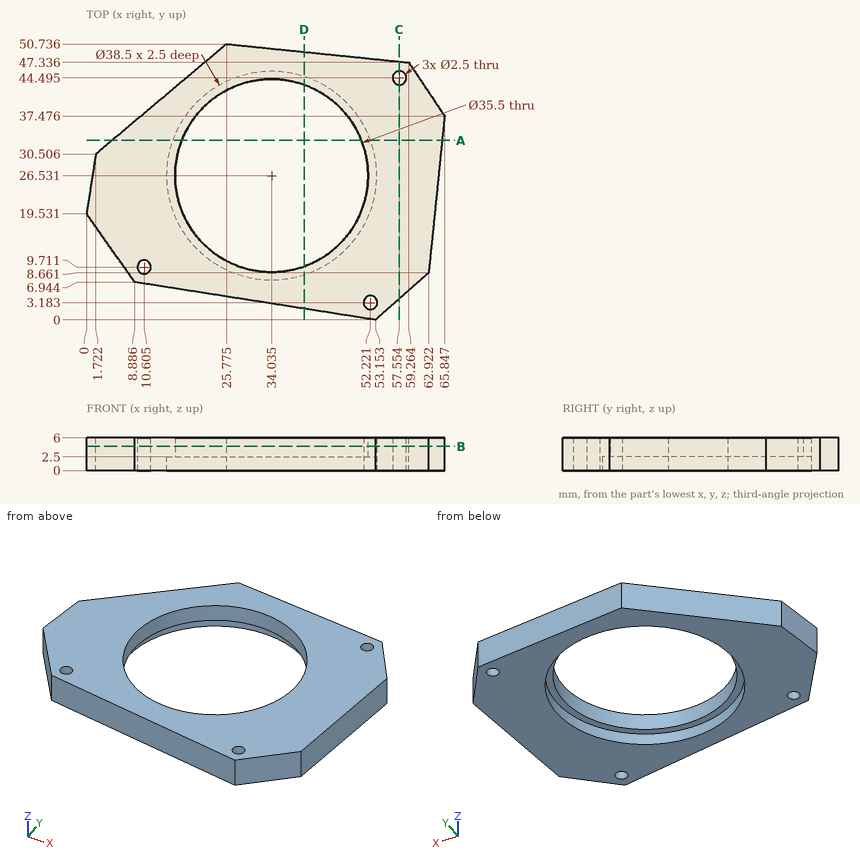
Geometry check sheet. Reference: drawing and pictorial views, mm from the part's lowest x, y, z. Give positions to 0.01 mm unless a question says otherwise; leave off trailing zeros. Order: outer loops, then holes, each group sorted by start corner. A loop starts at its lowest first (then second) coordinate and runs counter-clockwise, first axis right, second up. Notation, with made-up numbers: M 64.25,32 L 98.25,32 A23 ccw 98.25,67 Z; hole C 62.5,-17 d9. An arc over 180 degrees is marked long. Answer as CSV lines item,"result". Start each with the question number.
Item 1: Cross-section at B-B on z = 4.45. State how many separate pieces and enclosed holes the cut face has, plus the area to 3 significant figures.
Item 2: Gauge pin test, flat ends, axial feed: P1, Ø3, axis at x = 52.22, y = 3.18, coming from the -Z side; P2, Ø1.5, axis at x = 36, y = 43, coming from the -Z side; P3, Ø3, axis at x = 25, z = 5, coming from the -Y side. Record the tip position at first contact, or that the pin passes through.
Item 3: Cross-section at C-C on x = 57.5. Enter the section's corners in (y, z) (1 decimal), plus the area to 3 significant figures.
Item 4: Cross-section at D-D on x = 40. Enter the section's corners in (y, z).
Item 5: Cross-section at A-A on y = 33. Enter the section's corners in (x, z) (1 decimal), plus the area to 3 significant figures.
Item 6: Thickness scan on line 1 (Y direction, x = 24, z = 2) (1 decimal); line 2 (X direction, y = 10.5, z = 2.4) (1 decimal); line 3 (Y direction, x = 52, z = 2.8) (1 decimal). Record the ranges inside material, lowest first. Write a range as [from, to].
Established:
1,separate pieces,"1"
1,enclosed holes,"4"
1,area,"1,560 mm^2"
2,P1,"stops at z = 0"
2,P2,"passes through"
2,P3,"stops at y = 4.18"
3,outline,"M 3.9,0 L 43.2,0 L 43.2,6 L 3.9,6 Z; M 45.7,0 L 47.5,0 L 47.5,6 L 45.7,6 Z"
3,area,"247 mm^2"
4,outline,"M 2.06,0 L 8.23,0 L 8.23,2.5 L 9.81,2.5 L 9.81,6 L 2.06,6 Z; M 43.25,2.5 L 44.83,2.5 L 44.83,0 L 49.29,0 L 49.29,6 L 43.25,6 Z"
5,outline,"M 4.7,0 L 15.9,0 L 15.9,2.5 L 17.5,2.5 L 17.5,6 L 4.7,6 Z; M 50.6,2.5 L 52.2,2.5 L 52.2,0 L 65.4,0 L 65.4,6 L 50.6,6 Z"
5,area,"158 mm^2"
6,line 1,"y = [4.6, 10.1], [43, 49.2]"
6,line 2,"x = [6.4, 9.6], [11.6, 23.4], [44.7, 63.1]"
6,line 3,"y = [0.2, 2], [4.4, 48.1]"
